Here's how the part is built. I have some questions about the finished solid (model axes, mm). A direction names the side the tool comes from. Round coordinates to 2 decimals unless told otherwise and drop trailing zeros. Order: outer loops, then holes, each group sorted by start corner. A loop starts at its lowest first (then second) coordinate and runs counter-clockwise, first axis right, second up. Notation, with made-up numbers: M -11,14 L 47,14 A23 ccw 47,30 Z; hole C 29,-31.75 d10. An arc over 180 degrees is marked long. Use one line per item in the form item = value. Start each with the question number.
```python
from build123d import *

# Parameters (mm, degrees)
SKETCH1_R           = 8.5
BOSS_EXTRUDE1_DEPTH = 6
SKETCH2_R           = 2.5
BOSS_EXTRUDE2_DEPTH = 22
SKETCH3_R           = 3
CUT_EXTRUDE1_DEPTH  = 13
FILLET1_R           = 0.5


with BuildPart() as part:
    # Sketch1 → Boss-Extrude1 (new body)
    with BuildSketch(Plane(origin=(0, 0, 0), x_dir=(1, 0, 0), z_dir=(0, 1, 0))):
        with Locations(Location((0, 0, 0), (0, 0, 270))):
            Circle(SKETCH1_R)
    extrude(amount=BOSS_EXTRUDE1_DEPTH)

    # Sketch2 → Boss-Extrude2 (add)
    with BuildSketch(Plane(origin=(0, 6, 0), x_dir=(1, 0, 0), z_dir=(0, 1, 0))):
        with Locations(Location((0, 0, 0), (0, 0, 270))):
            Circle(SKETCH2_R)
    extrude(amount=BOSS_EXTRUDE2_DEPTH)

    # Sketch3 → Cut-Extrude1 (cut)
    with BuildSketch(Plane(origin=(0, 6, 0), x_dir=(1, 0, 0), z_dir=(0, 1, 0))):
        with Locations((-8.5, 0)):
            Circle(SKETCH3_R)
        with Locations((0, 8.5)):
            Circle(SKETCH3_R)
        with Locations((8.5, 0)):
            Circle(SKETCH3_R)
        with Locations((0, -8.5)):
            Circle(SKETCH3_R)
    extrude(amount=-CUT_EXTRUDE1_DEPTH, mode=Mode.SUBTRACT)

    # Fillet1
    fillet1_edges = [part.edges().sort_by_distance(p)[0] for p in [
        (-7.970588235, 3, -2.952917741),
        (-7.970588235, 3, 2.952917741),
        (2.952917741, 3, -7.970588235),
        (-2.952917741, 3, -7.970588235),
        (7.970588235, 3, 2.952917741),
        (7.970588235, 3, -2.952917741),
        (-2.952917741, 3, 7.970588235),
        (2.952917741, 3, 7.970588235),
    ]]
    fillet(fillet1_edges, radius=FILLET1_R)


solid = part.part
```
1) On a 3-axis mill with a long thin cutter (end or side, diameter ignored), from which of +Z, -Z, +X, -X, +Y, -Y can I reach the whole of each face in a straight line? I mean faces 1 (the cylindrical face through (-5.5, 3, 0.1)), 2 (the flat face through (2, 6, -2)). Say none if no direction works.
2) If we section it at B-B on z = 0: Write out the boundary of the cut face in (x, y), then the cut area to 3 significant figures.
3) If we section it at C-C on z = -6: Write out the boundary of the cut face in (x, y), then the cut area to 3 significant figures.
4) Will these pins go through, and if not, where does the flat tip stop? pin 1 Ø1.5 at (x, y) = (-2, 19.5) entering from +Z; pin 2 Ø1.5 at (y, z) = (5.5, 6) entering from +X; pin 3 Ø3 at (x, y) = (-1, 10.5) entering from +Z.
5) If we mould it in two halves opening along X, with no side actions, what happens to faces 3 (the cylindrical face through (-6.04, 2.96, 5.98)), 4 (the cylindrical face through (0.1, 3, 5.5)), 5 (the cylindrical face through (6.04, 2.96, -5.98)), 6 (the cylindrical face through (-0.1, 3, -5.5))? For each: +X half, -X half, draft (parallel to the pull), parting line (faces both ways), or undercut.
6) If we section it at D-D on y = 19.5: Write out the boundary of the cut face in (x, z), then the cut area to 3 significant figures.
7) If I drill on line 1 (Y direction, x = -5.75, z = 3.25); line 2 (Z direction, x = -7, y = 1.5); line 3 (Z direction, x = 2, y = 9.75), over which ranges is the centre line in solid material (lowest first)?
8) If we section it at A-A on x = 0: Write out the boundary of the cut face in (y, z).
Completed:
q1.face_1 = -X, +Y, -Y
q1.face_2 = +Y
q2.outline = M -5.5,0 L 5.5,0 L 5.5,6 L 2.5,6 L 2.5,28 L -2.5,28 L -2.5,6 L -5.5,6 Z
q2.area = 176 mm²
q3.outline = M -6.02,0 L -1.66,0 L -1.66,6 L -6.02,6 Z; M 1.66,0 L 6.02,0 L 6.02,6 L 1.66,6 Z
q3.area = 52.3 mm²
q4.pin_1 = 2.17
q4.pin_2 = 6.68
q4.pin_3 = 2.5
q5.face_3 = -X half
q5.face_4 = undercut
q5.face_5 = +X half
q5.face_6 = undercut
q6.outline = C 0,0 d5
q6.area = 19.6 mm²
q7.line_1 = 0 to 6
q7.line_2 = -4.82 to -2.6, 2.6 to 4.82
q7.line_3 = -1.5 to 1.5
q8.outline = M 0,-5.5 L 6,-5.5 L 6,-2.5 L 28,-2.5 L 28,2.5 L 6,2.5 L 6,5.5 L 0,5.5 Z
